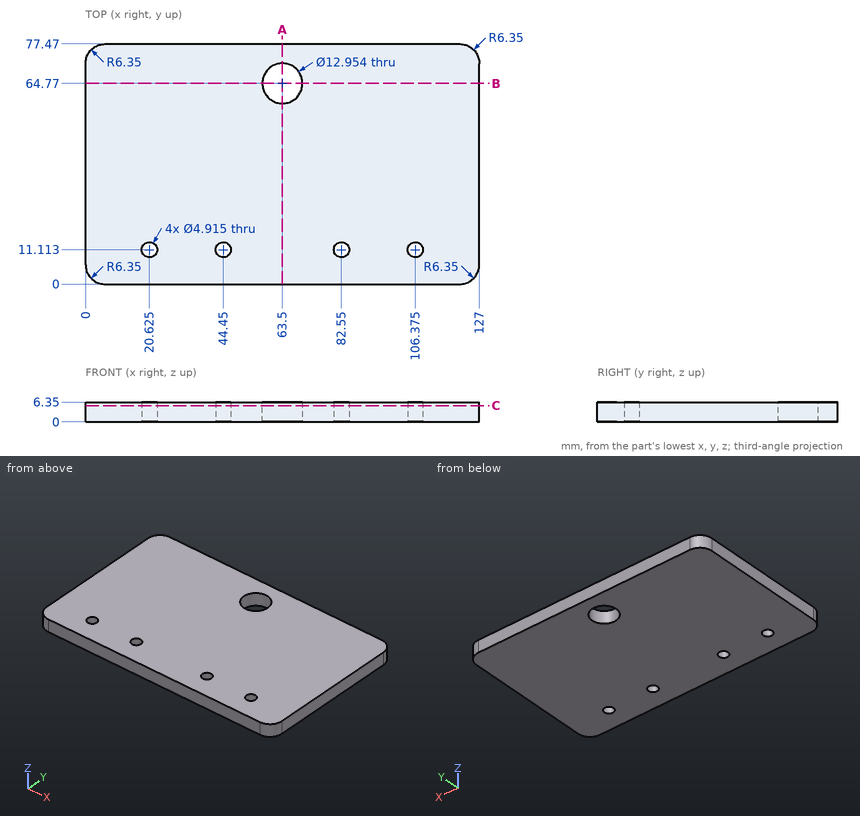
The figure shows three views and two pictorial views of one solid part (mm, origin at its lowest corner). Answer the questions. Round coordinates to 2 decimals unless told otherwise and drop trailing zeros. Order: outer loops, then holes, each group sorted by start corner. A loop starts at its lowest first (then second) coordinate and runs counter-clockwise, first axis right, second up. Notation, with made-up numbers: (-14.5, 28) - (31.5, 28) arc R27 ccw to (31.5, 62) - close; hole circle Ø6 at (-17, -17). An arc over 180 degrees is marked (long way). Write item = value, one per line. Start each with the question number.
1) Straight lines are drawn through the part: L1, parallel to X at y = 11.5, z = 3; L2, parallel to X at y = 64.5, z = 6; L3, parallel to Y at x = 82.55, z = 2 (1 decimal). For each, find the intervals that lie inside material, in ascending order.
2) Section B-B, the plane y = 64.77 is taken. Write down the section's boundary in (x, z), plus the area to 3 significant figures.
3) Section A-A, the plane x = 63.5 is taken. Write down the section's boundary in (y, z).
4) Section C-C, the plane z = 5.25 is taken. Count the separate pieces of the cut face and the enclosed holes in it, plus the area to 3 significant figures.
Results list:
q1.L1 = 0 to 18.2, 23.05 to 42.02, 46.88 to 80.12, 84.98 to 103.95, 108.8 to 127
q1.L2 = 0 to 57.03, 69.97 to 127
q1.L3 = 0 to 8.7, 13.6 to 77.5
q2.outline = (0, 0) - (57.02, 0) - (57.02, 6.35) - (0, 6.35) - close; (69.98, 0) - (127, 0) - (127, 6.35) - (69.98, 6.35) - close
q2.area = 724 mm^2
q3.outline = (0, 0) - (58.29, 0) - (58.29, 6.35) - (0, 6.35) - close; (71.25, 0) - (77.47, 0) - (77.47, 6.35) - (71.25, 6.35) - close
q4.separate_pieces = 1
q4.enclosed_holes = 5
q4.area = 9,600 mm^2
